Geometry: final body of the model. Coordinates: model frame, mm. Face numbers are marked on the shaded views. Give positions to 0.01 mm unless a question says otherwise; leave off trailing zeros. Loops run counter-clockwise (first coordinate to the right, second up) from the corner with the lowest first, then second, coordinate; pieces in that order, holes last. Notation, with made-up numbers: (2.5, 37.5) - (33.5, 37.5) arc R8 ccw to (33.5, 44.5) - close; hole circle Ø11 at (71, 56.5). An arc over 180 degrees is marked (long way). Use one line per item in the form item = value.
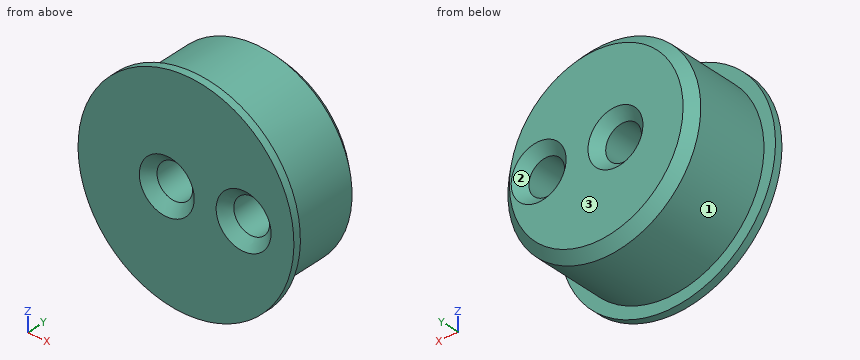
```python
from build123d import *
from build123d.topology import SkipClean

# Parameters (mm, degrees)
SKETCH_1_R      = 5.02
SKETCH_1_R_2    = 0.93
EXTRUDE_1_DEPTH = 4.4
EXTRUDE_START   = 0.4
SKETCH_3_R      = 5.62
SKETCH_3_R_2    = 0.93
EXTRUDE_2_DEPTH = 0.4
CHAMFER_1_SIZE  = 0.5


with BuildPart() as part:
    # Sketch 1 → Extrude 1 (new body)
    with BuildSketch(Plane(origin=(0, 0, 0), x_dir=(1, 0, 0), z_dir=(0, 1, 0))):
        with Locations(Location((0, 0, 0), (0, 0, 270))):
            Circle(SKETCH_1_R)
        with Locations(Location((3, 0, 0), (0, 0, 270))):
            Circle(SKETCH_1_R_2, mode=Mode.SUBTRACT)
        with Locations(Location((-1, 0, 0), (0, 0, 90))):
            Circle(SKETCH_1_R_2, mode=Mode.SUBTRACT)
    extrude(amount=EXTRUDE_1_DEPTH)

    # Sketch 3 → Extrude 2 (add)
    with SkipClean():  # the faces are left unmerged after this step: merging them gives an invalid solid
        with BuildSketch(Plane.XZ.offset(EXTRUDE_START)):
            with Locations(Location((0, 0, 0), (0, 0, 270))):
                Circle(SKETCH_3_R)
            with Locations(Location((3, 0, 0), (0, 0, 270))):
                Circle(SKETCH_3_R_2, mode=Mode.SUBTRACT)
            with Locations(Location((-1, 0, 0), (0, 0, 270))):
                Circle(SKETCH_3_R_2, mode=Mode.SUBTRACT)
        extrude(amount=-EXTRUDE_2_DEPTH)

    # Chamfer 1
    chamfer_1_edges = [part.edges().sort_by_distance(p)[0] for p in [
        (3, -0.4, 0.93),
        (-1, -0.4, 0.93),
        (0, 4.4, -5.02),
        (3, 4.4, -0.93),
        (-1, 4.4, 0.93),
    ]]
    chamfer(chamfer_1_edges, length=CHAMFER_1_SIZE)


solid = part.part
```
(1) Pull-direction query (Z, two-part tool) for the marked faces 1, 2 and 3; classes: released by +Z, released by -Z, zero draft, split by the parting line, or undercut.
Solution:
face_1 = split by the parting line
face_2 = undercut
face_3 = zero draft
(2) Pin query (flat end, axial travel): P1, Ø2, axis at y = 3, z = -1, coming from the +X side; P2, Ø1.5, axis at x = -1, z = 0, coming from the +Y side. Return the tip coordinate at first contact, or that it passes through.
Solution:
P1 = 5.02
P2 = through
(3) Material intervals for L1, parallel to X at y = 1.2, z = 0; L2, parallel to Y at x = 1, z = -5; L3, parallel to Z at x = 3, y = 1.65, sorted ascending. Write a range as from..to.
Solution:
L1 = -5.02..-1.93, -0.07..2.07, 3.93..5.02
L2 = -0.4..0
L3 = -4.02..-0.93, 0.93..4.02
(4) Cut plane B-B (y = 2.9). Return the cut outline in (x, z).
Solution:
outline = circle Ø10.04 at (0, 0); hole circle Ø1.86 at (-1, 0); hole circle Ø1.86 at (3, 0)
(5) Cut plane A-A (z = 0). Give the number of separate pieces and of enclosed holes in the cut face, plus the area to 3 significant figures.
Solution:
separate_pieces = 3
enclosed_holes = 0
area = 29.6 mm2
